```python
from build123d import *

# Parameters (mm, degrees)
F0_R      = 45
F1_DEPTH  = 25.5
F2_R      = 58
F3_DEPTH  = 1
F4_SIZE   = 8
F5_R      = 30
F6_DEPTH  = 6
F7_SIZE   = 5.99999
F9_R      = 11
F10_DEPTH = 25
F11_R     = 11
F11_R_2   = 10
F12_DEPTH = 5


# Not quite as in the source:
# - a fillet or chamfer is up to 0.001 mm smaller than in the source, because OpenCascade refuses the exact size


with BuildPart() as f1:
    # F0 (on Front) → F1 (new body)
    with BuildSketch(Plane.XZ):
        Circle(F0_R)
    extrude(amount=F1_DEPTH)

    # F2 (on face) → F3 (cut)
    with BuildSketch(Plane(origin=(0, 0, 0), x_dir=(-1, 0, 0), z_dir=(0, 1, 0))):
        Circle(F2_R)
    extrude(amount=-F3_DEPTH, mode=Mode.SUBTRACT)

    # F4
    f4_edges = [f1.edges().sort_by_distance(p)[0] for p in [
        (-45, -25.5, 0),
    ]]
    chamfer(f4_edges, length=F4_SIZE)

    # F5 (on face) → F6 (join)
    with BuildSketch(Plane.XZ.offset(25.5)):
        Circle(F5_R)
    extrude(amount=F6_DEPTH)

    # F7 (size 6 in the source; OpenCascade refuses exactly that, so slightly less here)
    f7_edges = [f1.edges().sort_by_distance(p)[0] for p in [
        (-30, -31.5, 0),
    ]]
    chamfer(f7_edges, length=F7_SIZE)

    # F9 (on face) → F10 (cut)
    with BuildSketch(Plane.XZ.offset(31.5)):
        Circle(F9_R)
    extrude(amount=-F10_DEPTH, mode=Mode.SUBTRACT)

    # F11 (on face) → F12 (join)
    with BuildSketch(Plane.XZ.offset(31.5)):
        Circle(F11_R)
        Circle(F11_R_2, mode=Mode.SUBTRACT)
    extrude(amount=-F12_DEPTH)


solid = f1.part
```
Input: part model. Units: mm. Frame: model coordinates. A direction names the side the tool comes from. Coordinates: 2 decimals unless noted, no trailing zeros. Loops run counter-clockwise (first coordinate to the right, second up) from the corner with the lowest first, then second, coordinate; pieces in that order, holes last. Notation, with made-up numbers: (76.25, 60) - (113.25, 60) arc R30 cw to (113.25, 83) - close; hole circle Ø3 at (-31.75, 50.5). An arc over 180 degrees is marked (long way). Answer in a Markdown table with one row per item.
(1) Material intervals for L1, parallel to Z at x = 0, y = -29; L2, parallel to Z at x = 0, y = -27.75; L3, parallel to Y at x = -11.5, z = -28, sorted ascending. Write a range as from..to.
Model answer:
| item | result |
|---|---|
| L1 | z = -26.5..-10, 10..26.5 |
| L2 | z = -27.75..-10, 10..27.75 |
| L3 | y = -25.5..-1 |
(2) Set-up query: faces 4 (the face through (-0.2, -25.5, 30.3)), 5 (the face through (20.765, -9.134, -39.923)), 6 (the face through (0, -6.5, 0)). Return all of +Z, -Z, +X, -X, +Y, -Y with unobstructed straight access to the full face (end or side cutting, diameter ignored); none if empty.
Model answer:
| item | result |
|---|---|
| face 4 | -Y |
| face 5 | +Y, -Y |
| face 6 | none |
(3) Mould query, pull axis Z, two halves, no side actions, for faces 1 (the face through (10.3, -31.5, 0.3)), 2 (the face through (-2.38, -16.64, -10.74)), 3 (the face through (-29.67, -25.11, -22.75)). Classes: pulls with the +Z half, pulls with the -Z half, needs draft (parallel to the pull), parting line crosses it, or undercut.
Model answer:
| item | result |
|---|---|
| face 1 | needs draft |
| face 2 | undercut |
| face 3 | parting line crosses it |
(4) Cut plane D-D on y = -5. Output: boundary loops of the cut face in (x, z), plus the area to 3 significant figures.
Model answer:
| item | result |
|---|---|
| outline | circle Ø90 at (0, 0) |
| area | 6,360 mm² |
(5) Cut plane C-C on y = -24. Output: boundary loops of the cut face in (x, z), plus the area to 3 significant figures.
Model answer:
| item | result |
|---|---|
| outline | circle Ø77 at (0, 0); hole circle Ø22 at (0, 0) |
| area | 4,280 mm² |
(6) Pin query (flat end, axial travel): P1, Ø2, axis at y = -23.5, z = -31.5, coming from the -X side; P2, Ø1, axis at x = -18.5, y = -21.5, coming from the +Z side; P3, Ø17.5, axis at x = 0, z = 0, coming from the -Y side. Return the tip coordinate at first contact, or that it passes through.
Model answer:
| item | result |
|---|---|
| P1 | stops at x = -25.08 |
| P2 | stops at z = 37.2 |
| P3 | stops at y = -6.5 |
